CAD build for the part. Positions are in the model's coordinates, mm. A direction names the side the tool comes from. Give positions to 0.01 mm unless a question says otherwise; leave off trailing zeros. Loops run counter-clockwise (first coordinate to the right, second up) from the corner with the lowest first, then second, coordinate; pieces in that order, holes last. Notation, with made-up numbers: (-15, 82) -> (11, 82) arc R22 cw to (11, 119) -> close; hole circle Ø9 at (-39, 71.5). An arc over 180 degrees is marked (long way). Use one line per item in the form item = value.
```python
from build123d import *

# Parameters (mm, degrees)
CROQUIS1_R              = 2
SALIENTE_EXTRUIR1_DEPTH = 5
CROQUIS2_R              = 5.75
CROQUIS2_R_2            = 7.5
CORTAR_EXTRUIR1_DEPTH   = 10


with BuildPart() as part:
    # Croquis1 → Saliente-Extruir1 (new body)
    with BuildSketch(Plane.XY):
        Polygon((0, 33.333333333), (5, 33.333333333), (5, 50), (52, 50), (52, 45), (104, 45), (104, 50), (156, 50), (156, 45), (208, 45), (208, 50), (255, 50), (255, 33.333333333), (260, 33.333333333), (260, 16.666666667), (255, 16.666666667), (255, 0), (208, 0), (208, 5), (156, 5), (156, 0), (104, 0), (104, 5), (52, 5), (52, 0), (5, 0), (5, 16.666666667), (0, 16.666666667), align=None)
        with Locations((16, 16)):
            Circle(CROQUIS1_R, mode=Mode.SUBTRACT)
        with Locations(Location((244, 16, 0), (0, 0, 180))):
            Circle(CROQUIS1_R, mode=Mode.SUBTRACT)
    extrude(amount=SALIENTE_EXTRUIR1_DEPTH)

    # Croquis2 → Cortar-Extruir1 (cut)
    with BuildSketch(Plane.XY.offset(5)):
        with Locations((210, 20)):
            Circle(CROQUIS2_R)
        with Locations((150.5, 21)):
            Circle(CROQUIS2_R_2)
    extrude(amount=-CORTAR_EXTRUIR1_DEPTH, mode=Mode.SUBTRACT)


solid = part.part
```
1. Cut at B-B, the plane x = 187. Write the cut outline in (y, z), then the cut area to 3 significant figures.
Result sheet:
outline = (5, 0) -> (45, 0) -> (45, 5) -> (5, 5) -> close
area = 200 mm^2
2. Cut at A-A, the plane z = 1.6. State how many separate pieces and enclosed holes the cut face has, then the cut area to 3 significant figures.
Result sheet:
separate_pieces = 1
enclosed_holes = 4
area = 11,300 mm^2
3. Drop flat-ended pins along their axis: P1, Ø1.5, axis at x = 256.5, z = 3.5, coming from the -Y side; P2, Ø1, axis at x = 94, y = 24, coming from the -Z side; P3, Ø1.5, axis at x = 190, z = 3, coming from the -Y side; P4, Ø2.5, axis at x = 2, z = 3.5, coming from the +Y side. Give the stop position or say it passes through.
Result sheet:
P1 = 16.67
P2 = 0
P3 = 5
P4 = 33.33
4. Mould opens along X. For faces 6 (the flat face through (5, 42, 2)), 7 (the flat face through (255, 42, 2)), 8 (the flat face through (3, 16.667, 2)), 9 (the flat face through (156, 48, 2)) say: pulls with the +X half, pulls with the -X half, needs draft (parallel to the pull), parting line crosses it, or undercut.
Result sheet:
face_6 = pulls with the -X half
face_7 = pulls with the +X half
face_8 = needs draft
face_9 = undercut
5. Drill centre lines: line 1 (Y direction, x = 244, z = 2.2); line 2 (Y direction, x = 150.5, z = 3.5); line 3 (Y direction, x = 86.5, z = 0.4). Where is each one in solid material? Low to high.
Result sheet:
line_1 = 0 to 14, 18 to 50
line_2 = 0 to 13.5, 28.5 to 50
line_3 = 5 to 45
6. Tool access for faces 1 (the flat face through (78, 45, 2)), 2 (the flat face through (208, 2, 2)), 3 (the flat face through (260, 25, 2)), 4 (the flat face through (29, 0, 2)), 5 (the flat face through (258, 16.667, 2)): list every direction of +Z, -Z, +X, -X, +Y, -Y with a clear straight run to the whole face (end or side of a thin tool).
Result sheet:
face_1 = +Z, -Z, +Y
face_2 = +Z, -Z, -Y
face_3 = +Z, -Z, +X, +Y, -Y
face_4 = +Z, -Z, +X, -X, -Y
face_5 = +Z, -Z, +X, -Y
